Geometry check sheet. Reference: the model listing, model coordinates, mm. A direction names the side the tool comes from. Give positions to 0.01 mm unless a question says otherwise; leave off trailing zeros. Order: outer loops, then holes, each group sorted by start corner. A loop starts at its lowest first (then second) coordinate and runs counter-clockwise, first axis right, second up. Notation, with made-up numbers: M 68,40.25 L 106,40.25 A24 cw 106,76.25 Z; hole C 76.25,48 d7. An arc over 180 degrees is marked long. Answer as CSV lines item,"result".
from build123d import *

# Parameters (mm, degrees)
EXTRUDE_1_DEPTH     = 65
SKETCH_2_R          = 3
CUT_EXTRUDE_1_DEPTH = 65
SKETCH_3_W          = 19.333072345
SKETCH_3_H          = 35
CUT_EXTRUDE_2_DEPTH = 32.5
SKETCH_4_R          = 3
CUT_EXTRUDE_3_DEPTH = 65


with BuildPart() as part:
    # 草图1 → 凸台-拉伸1 (new body)
    with BuildSketch(Plane.XY):
        with BuildLine():
            Line((-27.5, 4.75), (-27.5, 0))
            Line((-27.5, 0), (-9, 0))
            Line((-9, 0), (-6.189701831, 2.966425845))
            ThreePointArc((-6.189701831, 2.966425845), (6.974322263, 15.188482133), (-7.644442426, 4.75))
            Line((-7.644442426, 4.75), (-27.5, 4.75))
        make_face()
    extrude(amount=EXTRUDE_1_DEPTH)

    # 草图2 → 切除-拉伸1 (cut)
    with BuildSketch(Plane(origin=(0, 4.75, 0), x_dir=(1, 0, 0), z_dir=(0, 1, 0))):
        with Locations(Location((-19.5, -8.5, 0), (0, 0, 180))):
            Circle(SKETCH_2_R)
        with Locations(Location((-19.5, -56.5, 0), (0, 0, 270))):
            Circle(SKETCH_2_R)
    extrude(amount=-CUT_EXTRUDE_1_DEPTH, mode=Mode.SUBTRACT)

    # 草图3 → 切除-拉伸2 (cut, symmetric)
    with BuildSketch(Plane(origin=(0, 4.75, 0), x_dir=(1, 0, 0), z_dir=(0, 1, 0))):
        with Locations((0.666536173, -32.5)):
            Rectangle(SKETCH_3_W, SKETCH_3_H)
    extrude(amount=CUT_EXTRUDE_2_DEPTH, both=True, mode=Mode.SUBTRACT)

    # 草图4 → 切除-拉伸3 (cut)
    with BuildSketch(Plane.XY.offset(65)):
        with Locations((0, 9.5)):
            Circle(SKETCH_4_R)
    extrude(amount=-CUT_EXTRUDE_3_DEPTH, mode=Mode.SUBTRACT)


solid = part.part
(1) Draft check along X on faces 1 (the face through (-2, 7, 50)), 2 (the face through (-9, 2, 33)), 3 (the face through (-27.5, 2, 32)), 4 (the face through (-7.615, 1.462, 57.395)). Enter one of: +X half, -X half, draft (parallel to the pull), parting line (faces both ways), or undercut.
The answers:
face 1,"draft"
face 2,"+X half"
face 3,"-X half"
face 4,"undercut"
(2) Gauge pin test, flat ends, axial feed: P1, Ø7, axis at x = -19.5, z = 8.5, coming from the -Y side; P2, Ø8, axis at x = -19.5, z = 56.5, coming from the +Y side; P3, Ø8, axis at y = 11.5, z = 54, coming from the -X side; P4, Ø1.4, axis at y = 2.5, z = 39, coming from the +X side. Record the tip position at first contact, or that the pin passes through.
The answers:
P1,"stops at y = 0"
P2,"stops at y = 4.75"
P3,"stops at x = -9"
P4,"stops at x = -9"
(3) Section check C-C on y = 16. Enter the section's corners in (x, z), then the cut area to 3 significant figures.
The answers:
outline,"M -6.22,0 L 6.22,0 L 6.22,15 L -6.22,15 Z; M -6.22,50 L 6.22,50 L 6.22,65 L -6.22,65 Z"
area,"373 mm2"
(4) Section check B-B on x = 0. Enter the section's corners in (y, z).
The answers:
outline,"M 0.5,0 L 6.5,0 L 6.5,15 L 0.5,15 Z; M 0.5,50 L 6.5,50 L 6.5,65 L 0.5,65 Z; M 12.5,0 L 18.5,0 L 18.5,15 L 12.5,15 Z; M 12.5,50 L 18.5,50 L 18.5,65 L 12.5,65 Z"
(5) Section check D-D on x = -19.5. Enter the section's corners in (y, z).
The answers:
outline,"M 0,0 L 4.75,0 L 4.75,5.5 L 0,5.5 Z; M 0,11.5 L 4.75,11.5 L 4.75,53.5 L 0,53.5 Z; M 0,59.5 L 4.75,59.5 L 4.75,65 L 0,65 Z"
(6) Tool access check on faces 5 (the face through (-7.615, 1.462, 7.395)), 6 (the face through (-5, 7, 0)), 7 (the face through (-2, 7, 15)). Record the directions out of +Z, -Z, +X, -X, +Y, -Y that give a thin tool (end or side, any length) a straight path to the whole face; none if there is none.
The answers:
face 5,"+Z, -Z, -Y"
face 6,"-Z, +X, -X, +Y, -Y"
face 7,"+X, +Y, -Y"
(7) Section check A-A on z = 8.5. Enter the section's corners in (x, y), then the cut area to 3 significant figures.
The answers:
outline,"M -27.5,0 L -22.5,0 L -22.5,4.75 L -27.5,4.75 Z; M -16.5,0 L -9,0 L -6.19,2.97 A9 ccw long -7.64,4.75 L -16.5,4.75 Z; hole C 0,9.5 d6"
area,"293 mm2"
(8) Material ranges on line 1 (Y direction, x = 0, z = 56); line 2 (Z direction, x = -3.5, y = 12.5); line 3 (X direction, y = 1, z = 27.5), recorded low to high.
The answers:
line 1,"y = 0.5 to 6.5, 12.5 to 18.5"
line 2,"z = 0 to 15, 50 to 65"
line 3,"x = -27.5 to -9"
